Model file for the job. Use its own axes, mm. Coordinates: 2 decimals unless noted, no trailing zeros. Loops run counter-clockwise (first coordinate to the right, second up) from the corner with the lowest first, then second, coordinate; pieces in that order, holes last.
Autodesk Inventor part; units mm, degrees
ref_plane "YZ Plane" through (0, 0, 0) normal (1, 0, 0) x (0, 1, 0)
ref_plane "XZ Plane" through (0, 0, 0) normal (0, 1, 0) x (-1, 0, 0)
ref_plane "XY Plane" through (0, 0, 0) normal (0, 0, 1) x (1, 0, 0)
sketch "Skizze1" plane through (0, 0, 0) normal (0, 0, 1) x (1, 0, 0)
  line L0 (0, 0) -> (12, 0)
  line L1 (12, 0) -> (12, 8)
  line L2 (12, 8) -> (0, 8)
  line L3 (0, 8) -> (0, 0)
extrude "Extrusion1" add sketch "Skizze1" along normal blind 80
sketch "Skizze2" plane through (0, 0, 0) normal (0, 1, 0) x (-1, 0, 0)
  circle A0 centre (0, 70) radius 4.25
extrude "Extrusion2" cut sketch "Skizze2" along normal mid plane 20
properties part number "Stuetze"
Q1. Drill centre lines: line 1 (Z direction, x = 0.5, y = 3); line 2 (Z direction, x = 1.25, y = 3); line 3 (X direction, y = 5.5, z = 67). Where is each one in solid material? Low to high.
Answers:
line 1: z = 0 to 65.78, 74.22 to 80
line 2: z = 0 to 65.94, 74.06 to 80
line 3: x = 3.01 to 12
Q2. Slice it at C-C (z = 70). List the corners of the cut face in (x, y).
Answers:
outline: (4.25, 0) - (12, 0) - (12, 8) - (4.25, 8) - close
Q3. Mould opens along Z. For faces 1 (the flat face through (6, 4, 80)), 2 (the cylindrical face through (4.25, 3.94, 69.91)), 3 (the flat face through (6, 4, 0)), 4 (the flat face through (0, 4, 77)) say: +Z half, -Z half, draft (parallel to the pull), parting line (faces both ways), or undercut.
Answers:
face 1: +Z half
face 2: undercut
face 3: -Z half
face 4: draft
Q4. Slice it at A-A (x = 1.5). List the corners of the cut face in (y, z).
Answers:
outline: (0, 0) - (8, 0) - (8, 66.02) - (0, 66.02) - close; (0, 73.98) - (8, 73.98) - (8, 80) - (0, 80) - close
Q5. Flat gauge pin, fed straight in: P1, Ø4, axis at x = 3, z = 11, coming from the -Y side. Where does the tip first touch, or does it go through?
Answers:
P1: stops at y = 0
Q6. Slice it at B-B (y = 6.5). List the corners of the cut face in (x, z), and give its area (3 significant figures).
Answers:
outline: (0, 0) - (12, 0) - (12, 80) - (0, 80) - (0, 74.25) arc R4.25 cw to (0, 65.75) - close
area: 932 mm2
